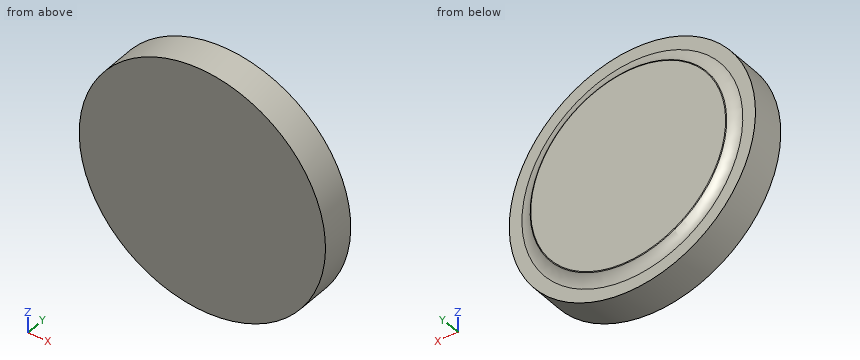
```python
from build123d import *

# Parameters (mm, degrees)
SKETCH_1_R      = 11
EXTRUDE_1_DEPTH = 3
SKETCH_2_R      = 8.75
EXTRUDE_2_DEPTH = 0.5
FILLET_1_R      = 1.5
FILLET_2_R      = 0.1


with BuildPart() as part:
    # 草图1 → 凸台-拉伸1 (new body)
    with BuildSketch(Plane(origin=(0, 0, 0), x_dir=(1, 0, 0), z_dir=(0, 1, 0))):
        with Locations(Location((0, 0, 0), (0, 0, 270))):
            Circle(SKETCH_1_R)
    extrude(amount=EXTRUDE_1_DEPTH)

    # 草图2 → 凸台-拉伸2 (add)
    with BuildSketch(Plane(origin=(0, 3, 0), x_dir=(1, 0, 0), z_dir=(0, 1, 0))):
        with Locations(Location((0, 0, 0), (0, 0, 270))):
            Circle(SKETCH_2_R)
    extrude(amount=EXTRUDE_2_DEPTH)

    # 圆角1
    # the kernel refuses this fillet: 1.5 mm, written as the material it adds along each edge
    with BuildSketch(Plane(origin=(0, 3, 0), x_dir=(0, 0, 1), z_dir=(-1, 0, 0))) as fillet_1_piece_1:
        with BuildLine():
            CenterArc((9.868033989, 1.5), FILLET_1_R, 221.810314896, 48.189685104)
            Line((8.75, 0.5), (8.72763932, 0.48))
            ThreePointArc((8.72763932, 0.48), (8.72, 0.25), (8.72, 0))
            Line((8.72, 0), (8.75, -0.03))
            Line((8.75, -0.03), (9.868033989, -0.03))
            Line((9.868033989, -0.03), (9.868033989, 0))
        make_face()
    revolve(axis=Axis((0, 3, 0), (0, 1, 0)))

    # 圆角2
    fillet_2_edges = [part.edges().sort_by_distance(p)[0] for p in [
        (0, 3.5, -8.75),
    ]]
    fillet(fillet_2_edges, radius=FILLET_2_R)


solid = part.part
```
Here's how the part is built. I have some questions about the finished solid (model axes, mm). Give positions to 0.01 mm unless a question says otherwise; leave off trailing zeros. Order: outer loops, then holes, each group sorted by start corner. A loop starts at its lowest first (then second) coordinate and runs counter-clockwise, first axis right, second up. Notation, with made-up numbers: M 21.25,22.25 L 27.25,22.25 A20 ccw 27.25,44.25 Z; hole C 3,4.25 d2. An arc over 180 degrees is marked long. Use a Markdown table: item, result. Add a question column.
1. Suppose I cut it at A-A (y = 1.15). List the corners of the cut face in (x, z) for me, and give its area (3 significant figures).
2. I need wall thicknesses on probe 1 along Y at (x, z) = (6.5, 7.5); probe 2 along X at (y, z) = (1.35, 7); probe 3 along Z at (x, y) = (2, 0.7). Which ranges of each line are inside material? Lowest first, please. Write a range as from..to.
3. For pin 1 Ø1 at (y, z) = (0.5, -2) entering from +X, with a flat end and sliding along its axis, tell me the tip position at first contact or that it passes through.
Results list:
| question | item | result |
|---|---|---|
| 1 | outline | C 0,0 d22 |
| 1 | area | 380 mm² |
| 2 | probe 1 | y = 0..3 |
| 2 | probe 2 | x = -8.49..8.49 |
| 2 | probe 3 | z = -10.82..10.82 |
| 3 | pin 1 | stops at x = 10.9 |
